Verification items for the finished model (mm, model axes). A direction names the side the tool comes from. Coordinates: 2 decimals unless noted, no trailing zeros. Order: outer loops, then holes, each group sorted by start corner. A loop starts at its lowest first (then second) coordinate and runs counter-clockwise, first axis right, second up.
Q1. Thickness scan on line 1 (Z direction, x = -0.4, y = 0.3); line 2 (Z direction, x = 0.9, y = 1.55); line 3 (Y direction, x = -0.25, z = -4.25). Record the ranges inside material, lowest first.
Q2. Depth check by flat-ended pin: P1, Ø1.5, axis at y = 1.5, z = -6.5, coming from the +X side. Enter the tip coordinate at first touch or a pass-through.
Q3. Cross-section at A-A, the plane y = 0. Record the boundary of the cut face in (x, z), and give its area (3 significant figures).
Q4. Cross-section at B-B, the plane z = -8.25. Record the boundary of the cut face in (x, y).
Q5. Set-up check for faces 1 (the flat face through (-1, -1, 2.35)), 2 (the cylindrical face through (-1.18, -0.26, -5.07)), 3 (the flat face through (-1, 0, 2)): record each of +Z, -Z, +X, -X, +Y, -Y from which the full face is reachable in a straight line by a thin tool's end or side.
from build123d import *

# Parameters (mm, degrees)
SCHNITT_LINEAR_AUSTRAGEN1_DEPTH = 1.5
FASE1_SIZE                      = 0.2
VERRUNDUNG1_R                   = 0.2
VERRUNDUNG2_R                   = 0.1


with BuildPart() as part:
    # Skizze1 → Rotation1 (revolve)
    with BuildSketch(Plane(origin=(0, 0, 0), x_dir=(0, 0, -1), z_dir=(1, 0, 0))):
        Polygon((-2.35, 0), (-2.35, 2.15), (0, 2.15), (0, 1.21), (10, 1.21), (10, 0), align=None)
    revolve(axis=Axis((0, 0, 21.919879518), (0, 0, -1)))

    # Skizze2 → Schnitt-Linear austragen1 (cut)
    with BuildSketch(Plane.XY.offset(2.35)):
        Polygon((1, -0.577350269), (1, 0.577350269), (0, 1.154700538), (-1, 0.577350269), (-1, -0.577350269), (0, -1.154700538), align=None)
    extrude(amount=-SCHNITT_LINEAR_AUSTRAGEN1_DEPTH, mode=Mode.SUBTRACT)

    # Fase1
    fase1_edges = [part.edges().sort_by_distance(p)[0] for p in [
        (0, -1.21, -10),
        (0, -2.15, 0),
        (0, -2.15, 2.35),
    ]]
    chamfer(fase1_edges, length=FASE1_SIZE)

    # Verrundung1
    verrundung1_edges = [part.edges().sort_by_distance(p)[0] for p in [
        (0.5, -0.866025404, 0.85),
        (1, -0.577350269, 1.6),
        (-0.5, -0.866025404, 0.85),
        (0, -1.154700538, 1.6),
        (-1, 0, 0.85),
        (-1, -0.577350269, 1.6),
        (-0.5, 0.866025404, 0.85),
        (-1, 0.577350269, 1.6),
        (0.5, 0.866025404, 0.85),
        (0, 1.154700538, 1.6),
        (1, 0, 0.85),
        (1, 0.577350269, 1.6),
        (0, -1.21, 0),
    ]]
    fillet(verrundung1_edges, radius=VERRUNDUNG1_R)

    # Verrundung2
    verrundung2_edges = [part.edges().sort_by_distance(p)[0] for p in [
        (-0.5, -0.866025404, 2.35),
        (-1, 0, 2.35),
        (-0.5, 0.866025404, 2.35),
        (0.5, 0.866025404, 2.35),
        (1, 0, 2.35),
        (0.5, -0.866025404, 2.35),
        (-0.973205081, -0.561880215, 2.35),
        (0, -1.123760431, 2.35),
        (0.973205081, -0.561880215, 2.35),
        (0.973205081, 0.561880215, 2.35),
        (0, 1.123760431, 2.35),
        (-0.973205081, 0.561880215, 2.35),
    ]]
    fillet(verrundung2_edges, radius=VERRUNDUNG2_R)


solid = part.part
Check values:
1. line 1: z = -10 to 0.85
1. line 2: z = 0 to 2.35
1. line 3: y = -1.18 to 1.18
2. P1: stops at x = 0.95
3. outline: (-2.15, 0.2) - (-1.95, 0) - (-1.41, 0) arc R0.2 cw to (-1.21, -0.2) - (-1.21, -9.8) - (-1.01, -10) - (1.01, -10) - (1.21, -9.8) - (1.21, -0.2) arc R0.2 cw to (1.41, 0) - (1.95, 0) - (2.15, 0.2) - (2.15, 2.15) - (1.95, 2.35) - (1.1, 2.35) arc R0.1 ccw to (1, 2.25) - (1, 1.05) arc R0.2 cw to (0.8, 0.85) - (-0.8, 0.85) arc R0.2 cw to (-1, 1.05) - (-1, 2.25) arc R0.1 ccw to (-1.1, 2.35) - (-1.95, 2.35) - (-2.15, 2.15) - close
3. area: 31.2 mm2
4. outline: circle Ø2.42 at (0, 0)
5. face 1: +Z, +X, -X, +Y, -Y
5. face 2: -Z
5. face 3: +Z
